Work out the finished part from the listing and answer in its coordinate system (mm). A direction names the side the tool comes from. Coordinates: 2 decimals unless noted, no trailing zeros. Order: outer loops, then holes, each group sorted by start corner. A loop starts at its lowest first (then second) coordinate and runs counter-clockwise, first axis right, second up. Notation, with made-up numbers: (-38.5, 31.5) - (2.5, 31.5) arc R17 ccw to (2.5, 46.5) - close; hole circle Ø4 at (53, -3.5). An arc over 180 degrees is marked (long way). Answer as a JSON object with one key per item and string values. Group by question number.
1) Section B-B (x = 16.5) is taken. Give the vertices of the cut face in (y, z).
2) Section A-A (z = 2.55) is taken. Give the vertices of the cut face in (x, y), plus the area to 3 significant figures.
3) The mould has two halves that part along X. Classify faces 3 (the face through (-86.592, -6.673, 1.479)), 4 (the face through (-1, 13, 3)), 5 (the face through (-33.171, -42.676, 1.479)): released by +X, released by -X, zero draft, split by the parting line, or undercut.
4) A tool of negligible diameter and unlimited length cuts with its end or side. For faces 1 (the face through (85.993, -8.261, 1.479)), 2 (the face through (33.02, -42.28, 1.48)), from which of +Z, -Z, +X, -X, +Y, -Y can it reach the whole face along a straight path? Write none if from no direction.
5) Each of these flat-tipped pins is pushed along its axis until it touches: P1, Ø4, axis at x = -88.61, y = 25.09, coming from the -Z side; P2, Ø1, axis at x = -51, z = 1.5, coming from the -Y side. Where does it stop, or does it pass through?
6) Section C-C (y = 44) is taken. Give the vertices of the cut face in (x, z).
7) Find the intervals of material crossed by line 1 along Y through (x, z) = (-13, 0.95); line 2 along X through (y, z) = (-50, 0.35); line 3 along X through (y, z) = (-47, 1.95), in increasing order.
from build123d import *

# Parameters (mm, degrees)
CROQUIS1_R              = 1.5
SALIENTE_EXTRUIR1_DEPTH = 3


with BuildPart() as part:
    # Croquis1 → Saliente-Extruir1 (new body)
    with BuildSketch(Plane.XY):
        with BuildLine():
            Line((87.218748359, 55.090741804), (-87.218748359, 55.090741804))
            ThreePointArc((-87.218748359, 55.090741804), (-86.279970689, -7.51104838), (-45.585521295, -55.090741804))
            Line((-45.585521295, -55.090741804), (-20.404037688, -29.909258196))
            Line((-20.404037688, -29.909258196), (20.648831544, -29.909258196))
            Line((20.648831544, -29.909258196), (45.741459084, -55.001885736))
            ThreePointArc((45.741459084, -55.001885736), (86.311649564, -7.427087381), (87.218748359, 55.090741804))
        make_face()
        with Locations((0, -24.909258196)):
            Circle(CROQUIS1_R, mode=Mode.SUBTRACT)
        with Locations((88.605744965, 25.090741804)):
            Circle(CROQUIS1_R, mode=Mode.SUBTRACT)
        with Locations((0, 25.090741804)):
            Circle(CROQUIS1_R, mode=Mode.SUBTRACT)
        with Locations((-88.605744965, 25.090741804)):
            Circle(CROQUIS1_R, mode=Mode.SUBTRACT)
    extrude(amount=SALIENTE_EXTRUIR1_DEPTH)


solid = part.part
Report:
{
 "1": {"outline": "(-29.91, 0) - (55.09, 0) - (55.09, 3) - (-29.91, 3) - close"},
 "2": {"outline": "(-87.22, 55.09) arc R92.23 ccw to (-45.59, -55.09) - (-20.4, -29.91) - (20.65, -29.91) - (45.74, -55) arc R92.23 ccw to (87.22, 55.09) - close; hole circle Ø3 at (-88.61, 25.09); hole circle Ø3 at (0, -24.91); hole circle Ø3 at (0, 25.09); hole circle Ø3 at (88.61, 25.09)", "area": "16,400 mm²"},
 "3": {"face 3": "released by -X", "face 4": "zero draft", "face 5": "undercut"},
 "4": {"face 1": "+Z, -Z, +X", "face 2": "+Z, -Z, -Y"},
 "5": {"P1": "stops at z = 0", "P2": "stops at y = -52.09"},
 "6": {"outline": "(-90.27, 0) - (90.27, 0) - (90.27, 3) - (-90.27, 3) - close"},
 "7": {"line 1": "y = -29.91 to 55.09", "line 2": "x = -53.56 to -40.49, 40.74 to 53.56", "line 3": "x = -57.53 to -37.49, 37.74 to 57.53"}
}
